Here's how the part is built. I have some questions about the finished solid (model axes, mm). A direction names the side the tool comes from. Coordinates: 2 decimals unless noted, no trailing zeros. Order: outer loops, then holes, each group sorted by start corner. A loop starts at its lowest first (then second) coordinate and runs counter-clockwise, first axis right, second up. Notation, with made-up numbers: (58.25, 38.5) - (69.25, 38.5) arc R10 ccw to (69.25, 46.5) - close; hole circle Ø10 at (22, 11.5). An arc over 180 degrees is marked (long way). Use CSV: the item, a comma, the result in double quotes. Start each with the question number.
from build123d import *

# Parameters (mm, degrees)
BOSS_EXTRUDE1_DEPTH = 6.35
SKETCH2_W           = 5
SKETCH2_H           = 37.5
CUT_EXTRUDE1_DEPTH  = 5
SKETCH3_W           = 2
SKETCH3_H           = 2.75
CUT_EXTRUDE2_DEPTH  = 5
SKETCH4_W           = 20
SKETCH4_H           = 1
SKETCH4_W_2         = 9.5
BOSS_EXTRUDE2_DEPTH = 5
SKETCH5_R           = 1.25
CUT_EXTRUDE3_DEPTH  = 5
SKETCH6_R           = 1.25
CUT_EXTRUDE4_DEPTH  = 6
CHAMFER1_SIZE       = 0.6


with BuildPart() as part:
    # Sketch1 → Boss-Extrude1 (new body)
    with BuildSketch(Plane(origin=(0, 0, 0), x_dir=(1, 0, 0), z_dir=(0, 1, 0))):
        with BuildLine():
            Line((-46, -35), (46, -35))
            ThreePointArc((46, -35), (48.828427125, -33.828427125), (50, -31))
            Line((50, -31), (50, 31))
            ThreePointArc((50, 31), (48.828427125, 33.828427125), (46, 35))
            Line((46, 35), (-46, 35))
            ThreePointArc((-46, 35), (-48.828427125, 33.828427125), (-50, 31))
            Line((-50, 31), (-50, -31))
            ThreePointArc((-50, -31), (-48.828427125, -33.828427125), (-46, -35))
        make_face()
    extrude(amount=BOSS_EXTRUDE1_DEPTH)

    # Sketch2 → Cut-Extrude1 (cut)
    with BuildSketch(Plane.XZ):
        with Locations((-47.5, -5.25)):
            Rectangle(SKETCH2_W, SKETCH2_H)
    extrude(amount=-CUT_EXTRUDE1_DEPTH, mode=Mode.SUBTRACT)

    # Sketch3 → Cut-Extrude2 (cut)
    with BuildSketch(Plane.ZY.offset(50)):
        with Locations((-25, 1.975)):
            Rectangle(SKETCH3_W, SKETCH3_H)
        with Locations((14.5, 1.975)):
            Rectangle(SKETCH3_W, SKETCH3_H)
    extrude(amount=-CUT_EXTRUDE2_DEPTH, mode=Mode.SUBTRACT)

    # Sketch4 → Boss-Extrude2 (add)
    with BuildSketch(Plane.ZY.offset(45)):
        with Locations((-12, 2.5)):
            Rectangle(SKETCH4_W, SKETCH4_H)
        Polygon((-1, 3), (-2, 3), (-2, 2), (-2, 1.25), (-1, 1.25), align=None)
        Polygon((2, 2), (2, 3), (1, 3), (1, 1.25), (2, 1.25), align=None)
        with Locations((6.75, 2.5)):
            Rectangle(SKETCH4_W_2, SKETCH4_H)
    extrude(amount=BOSS_EXTRUDE2_DEPTH)

    # Sketch5 → Cut-Extrude3 (cut)
    with BuildSketch(Plane.XZ):
        with Locations(Location((-36, 30.86, 0), (0, 0, 270))):
            Circle(SKETCH5_R)
        with Locations(Location((40.6, 30.86, 0), (0, 0, 270))):
            Circle(SKETCH5_R)
        with Locations(Location((40.6, -30.86, 0), (0, 0, 270))):
            Circle(SKETCH5_R)
        with Locations(Location((-36, -30.86, 0), (0, 0, 270))):
            Circle(SKETCH5_R)
    extrude(amount=-CUT_EXTRUDE3_DEPTH, mode=Mode.SUBTRACT)

    # Sketch6 → Cut-Extrude4 (cut)
    with BuildSketch(Plane(origin=(0, 0, -35), x_dir=(-1, 0, 0), z_dir=(0, 0, -1))):
        with Locations((-40.6, 3)):
            Circle(SKETCH6_R)
        with Locations((36, 3)):
            Circle(SKETCH6_R)
    cut_extrude4 = extrude(amount=-CUT_EXTRUDE4_DEPTH, mode=Mode.SUBTRACT)

    # Mirror1: Cut-Extrude4 across plane
    add(cut_extrude4.mirror(Plane.XY), mode=Mode.SUBTRACT)

    # Chamfer1
    chamfer1_edges = [part.edges().sort_by_distance(p)[0] for p in [
        (48.828427125, 6.35, 33.828427125),
        (50, 6.35, 0),
        (48.828427125, 6.35, -33.828427125),
        (0, 6.35, -35),
        (-48.828427125, 6.35, -33.828427125),
        (-50, 6.35, 0),
        (-48.828427125, 6.35, 33.828427125),
        (0, 6.35, 35),
    ]]
    chamfer(chamfer1_edges, length=CHAMFER1_SIZE)


solid = part.part
Item 1: Suppose I cut it at A-A on x = -36. State how many separate pieces and enclosed holes the cut face has, then the cut area to 3 significant figures.
Item 2: Suppose I cut it at B-B on z = -4.5. Write out the boundary of the cut face in (x, y).
Item 3: Please list where these lines run through material, in increasing order: line 1 along X through (y, z) = (3, 29.85); line 2 along Z through (x, y) = (-36, 1); line 3 along X through (y, z) = (4.5, -0.5). Write a range as from..to.
Item 4: We'd pull the mould along Y, two halves only. Please class faces 1 (the flat face through (-1, 0, 0)), 2 (the cylindrical face through (-34.75, 3.05, -29.53)), 3 (the flat face through (-50, 5.4, 6.5)), 4 (the flat face through (-1, 6.35, 0)): released by +Y, released by -Y, zero draft, split by the parting line, or undercut.
Item 5: For pin 1 Ø1.4 at (x, y) = (-48, 2.5) entering from -Z; pin 2 Ø1.2 at (x, z) = (40.5, 31) entering from -Y; pin 3 Ø0.7 at (x, y) = (-47, 0.5) entering from -Z, each with a flat end and sliding along its axis, tell me the tip position at first contact or that it passes through.
Item 6: For faces 5 (the cylindrical face through (-34.946, 1.146, -31.532)), 6 (the flat face through (-47, 2, 7)), 7 (the flat face through (41, 3, -29)), 8 (the flat face through (-48, 0.6, 14)), which set-ups out of +Z, -Z, +X, -X, +Y, -Y let a thin tool reach every point of the face, with its end or its side?
Here are the results:
1,separate pieces,"3"
1,enclosed holes,"0"
1,area,"402 mm^2"
2,outline,"(-50, 2) - (-45, 2) - (-45, 0) - (50, 0) - (50, 5.75) - (49.4, 6.35) - (-49.4, 6.35) - (-50, 5.75) - (-50, 5) - (-45, 5) - (-45, 3) - (-50, 3) - close"
3,line 1,"-50..-37.25, -34.75..39.35, 41.85..50"
3,line 2,"-35..-32.11, -29.61..29.61, 32.11..35"
3,line 3,"-45..50"
4,face 1,"released by -Y"
4,face 2,"undercut"
4,face 3,"zero draft"
4,face 4,"released by +Y"
5,pin 1,"z = -34.78"
5,pin 2,"y = 5"
5,pin 3,"z = -34.95"
6,face 5,"-Y"
6,face 6,"-X, -Y"
6,face 7,"-Z"
6,face 8,"-X"
